Here's how the part is built. I have some questions about the finished solid (model axes, mm). A direction names the side the tool comes from. Give positions to 0.01 mm unless a question says otherwise; leave off trailing zeros. Write each loop counter-clockwise with the first axis right and the second up, starting at its lowest first coordinate (ties: lowest second). Pieces come first, ordered by that corner, then holes. Notation, with made-up numbers: (-5, 18.5) -> (48, 18.5) arc R14 ccw to (48, 34.5) -> close; hole circle Ø11 at (85, 74). An arc over 180 degrees is marked (long way). Return JSON: item names as keys, results as strings.
from build123d import *

# Parameters (mm, degrees)
BOSS_EXTRUDE1_DEPTH                  = 29.8
FILLET1_R                            = 0.5
F_8_2_8_2_DIAMETER_HOLE1_D           = 8.2
F_8_2_8_2_DIAMETER_HOLE1_CSINK_D     = 8.25
F_8_2_8_2_DIAMETER_HOLE1_CSINK_ANGLE = 90
M4_TAPPED_HOLE1_D                    = 3.3
M4_TAPPED_HOLE1_CSINK_D              = 4.05
M4_TAPPED_HOLE1_CSINK_ANGLE          = 90


with BuildPart() as part:
    # Sketch1 → Boss-Extrude1 (new body)
    with BuildSketch(Plane.XY):
        Polygon((-3.5, 4), (3.5, 4), (7.5, 0), (15.35, 0), (15.35, -10.9), (16.9, -12.45), (16.9, -18), (8.9, -18), (7.9, -16.8), (-7.9, -16.8), (-8.9, -18), (-16.9, -18), (-16.9, -12.45), (-15.35, -10.9), (-15.35, 0), (-7.5, 0), align=None)
    extrude(amount=BOSS_EXTRUDE1_DEPTH)

    # Fillet1
    fillet1_edges = [part.edges().sort_by_distance(p)[0] for p in [
        (-5.5, 2, 29.8),
        (11.425, 0, 0),
        (15.35, -5.45, 0),
        (16.125, -11.675, 0),
        (-11.425, 0, 29.8),
        (16.9, -15.225, 0),
        (12.9, -18, 0),
        (8.4, -17.4, 0),
        (0, -16.8, 0),
        (-8.4, -17.4, 0),
        (-12.9, -18, 0),
        (-16.9, -15.225, 0),
        (-16.125, -11.675, 0),
        (-15.35, -5.45, 0),
        (-11.425, 0, 0),
        (-15.35, -5.45, 29.8),
        (-5.5, 2, 0),
        (0, 4, 0),
        (5.5, 2, 0),
        (-16.125, -11.675, 29.8),
        (7.5, 0, 14.9),
        (15.35, 0, 14.9),
        (15.35, -10.9, 14.9),
        (16.9, -12.45, 14.9),
        (16.9, -18, 14.9),
        (8.9, -18, 14.9),
        (7.9, -16.8, 14.9),
        (-7.9, -16.8, 14.9),
        (-8.9, -18, 14.9),
        (-16.9, -18, 14.9),
        (-16.9, -12.45, 14.9),
        (-15.35, -10.9, 14.9),
        (-15.35, 0, 14.9),
        (-7.5, 0, 14.9),
        (-3.5, 4, 14.9),
        (3.5, 4, 14.9),
        (-16.9, -15.225, 29.8),
        (-12.9, -18, 29.8),
        (-8.4, -17.4, 29.8),
        (0, -16.8, 29.8),
        (8.4, -17.4, 29.8),
        (12.9, -18, 29.8),
        (5.5, 2, 29.8),
        (16.9, -15.225, 29.8),
        (16.125, -11.675, 29.8),
        (15.35, -5.45, 29.8),
        (11.425, 0, 29.8),
        (0, 4, 29.8),
    ]]
    fillet(fillet1_edges, radius=FILLET1_R)

    # Ø8.2 (8.2) Diameter Hole1 (through all)
    with Locations(Plane(origin=(0, -7.513450587, 29.8), x_dir=(1, 0, 0), z_dir=(0, 0, 1))):
        with Locations((0, 0)):
            CounterSinkHole(F_8_2_8_2_DIAMETER_HOLE1_D / 2, F_8_2_8_2_DIAMETER_HOLE1_CSINK_D / 2, counter_sink_angle=F_8_2_8_2_DIAMETER_HOLE1_CSINK_ANGLE)

    # M4 Tapped Hole1 (through all)
    with Locations(Plane(origin=(11.9, -18, 24.4), x_dir=(0, 0, -1), z_dir=(0, -1, 0))):
        with Locations((0, 0), (19.4, 0), (19.4, -23.8), (0, -23.8)):
            CounterSinkHole(M4_TAPPED_HOLE1_D / 2, M4_TAPPED_HOLE1_CSINK_D / 2, counter_sink_angle=M4_TAPPED_HOLE1_CSINK_ANGLE)


solid = part.part
1. If I drill on line 1 (Z direction, x = 11.9, y = -13.5); line 2 (X direction, y = -7.5, z = 5); line 3 (X direction, y = -1.75, z = 5), over which ranges is the centre line in solid material (lowest first)? Write a range as [from, to].
Taken from the geometry:
{"line 1": "z = [0, 3.35], [6.65, 22.75], [26.05, 29.8]", "line 2": "x = [-15.35, -13.55], [-10.25, -4.1], [4.1, 10.25], [13.55, 15.35]", "line 3": "x = [-15.35, -13.55], [-10.25, 10.25], [13.55, 15.35]"}
2. Suppose I cut it at B-B, the plane x = 0. List the corners of the cut face in (y, z) for me (3 decimals).
Taken from the geometry:
{"outline": "(-16.8, 0.5) arc R0.5 ccw to (-16.3, 0) -> (-11.613, 0) -> (-11.613, 29.775) -> (-11.638, 29.8) -> (-16.3, 29.8) arc R0.5 ccw to (-16.8, 29.3) -> close; (-3.413, 0) -> (3.5, 0) arc R0.5 ccw to (4, 0.5) -> (4, 29.3) arc R0.5 ccw to (3.5, 29.8) -> (-3.388, 29.8) -> (-3.413, 29.775) -> close"}
3. Suppose I cut it at A-A, the plane x = -11.9. List the corners of the cut face in (y, z) for me (3 decimals).
Taken from the geometry:
{"outline": "(-18, 0.5) arc R0.5 ccw to (-17.5, 0) -> (-0.5, 0) arc R0.5 ccw to (0, 0.5) -> (0, 3.35) -> (-17.625, 3.35) -> (-18, 2.975) -> close; (-18, 7.025) -> (-17.625, 6.65) -> (0, 6.65) -> (0, 22.75) -> (-17.625, 22.75) -> (-18, 22.375) -> close; (-18, 26.425) -> (-17.625, 26.05) -> (0, 26.05) -> (0, 29.3) arc R0.5 ccw to (-0.5, 29.8) -> (-17.5, 29.8) arc R0.5 ccw to (-18, 29.3) -> close"}
4. If we mould it in two halves opening along Y, with no side actions, what happens to faces 6 (the face through (-11, 0, 15)), 7 (the face through (15.35, -6, 15)), 8 (the face through (8.5, -17.3, 29.65)), 9 (the face through (0.889, -11.516, 14.679))? For each: released by +Y, released by -Y, zero draft, split by the parting line, or undercut.
Taken from the geometry:
{"face 6": "released by +Y", "face 7": "zero draft", "face 8": "released by -Y", "face 9": "undercut"}
5. Suppose I cut it at D-D, the plane y = -8.25. Count the separate pieces of the cut face and the enclosed holes in it, and give its area (3 significant figures).
Taken from the geometry:
{"separate pieces": "2", "enclosed holes": "4", "area": "640 mm²"}
6. For pin 1 Ø3.5 at (x, z) = (11, 15) entering from +Y; pin 2 Ø8 at (x, z) = (9.5, 14) entering from +Y; pin 3 Ø1 at (y, z) = (-12, 4.5) entering from +X, each with a flat end and sliding along its axis, tell me the tip position at first contact or that it passes through.
Taken from the geometry:
{"pin 1": "stops at y = 0", "pin 2": "stops at y = 2", "pin 3": "stops at x = 16.87"}
7. Which directions (+Z, -Z, +X, -X, +Y, -Y) give clear straight access to the entire face, cutting with the end or side of a thin tool? Please do faces 1 (the face through (8.5, -17.3, 0.15)), 2 (the face through (4, -9, 0)), 3 (the face through (-8.4, -17.4, 14.7)), 4 (the face through (-16.02, -11.77, 29.65)), 5 (the face through (-15.35, -6, 15)).
Taken from the geometry:
{"face 1": "-Z, -Y", "face 2": "-Z, +X, -X, +Y, -Y", "face 3": "+Z, -Z, -Y", "face 4": "+Z, -X, +Y", "face 5": "+Z, -Z, -X, +Y"}
